Input: part model. Units: mm. Frame: model coordinates. A direction names the side the tool comes from. Give positions to 0.01 mm unless a question says otherwise; leave off trailing zeros. Loops run counter-clockwise (first coordinate to the right, second up) from the corner with the lowest first, then second, coordinate; pieces in that order, holes last. Notation, with made-up numbers: (52.25, 13.25) - (85.25, 13.25) arc R19 ccw to (85.25, 41.25) - close; hole circle Ø10 at (88, 59.5). An arc over 180 degrees is marked (long way). Answer as a JSON object with one key per item and string values.
from build123d import *

# Parameters (mm, degrees)
SKETCH1_W           = 25
SKETCH1_H           = 12
SKETCH1_R           = 1.5
BOSS_EXTRUDE1_DEPTH = 1
SKETCH2_R           = 1.5
SKETCH2_R_2         = 1
BOSS_EXTRUDE2_DEPTH = 6.25
BOSS_EXTRUDE3_START = 12.5
SKETCH3_R           = 1.5
SKETCH3_R_2         = 1
BOSS_EXTRUDE3_DEPTH = 6.25


with BuildPart() as part:
    # Sketch1 → Boss-Extrude1 (new body)
    with BuildSketch(Plane(origin=(0, 0, 0), x_dir=(1, 0, 0), z_dir=(0, 1, 0))):
        with Locations((12.5, 6)):
            Rectangle(SKETCH1_W, SKETCH1_H)
        with Locations((6, 6)):
            Circle(SKETCH1_R, mode=Mode.SUBTRACT)
        with Locations((19, 6)):
            Circle(SKETCH1_R, mode=Mode.SUBTRACT)
    extrude(amount=BOSS_EXTRUDE1_DEPTH)

    # Sketch2 → Boss-Extrude2 (add)
    with BuildSketch(Plane(origin=(0, 0, 0), x_dir=(0, 0, -1), z_dir=(1, 0, 0))):
        with Locations((-1, 1)):
            Circle(SKETCH2_R)
        with Locations((-1, 1)):
            Circle(SKETCH2_R_2, mode=Mode.SUBTRACT)
    extrude(amount=BOSS_EXTRUDE2_DEPTH)

    # Sketch3 → Boss-Extrude3 (add)
    with BuildSketch(Plane(origin=(0, 0, 0), x_dir=(0, 0, -1), z_dir=(1, 0, 0)).offset(BOSS_EXTRUDE3_START)):
        with Locations((-1, 1)):
            Circle(SKETCH3_R)
        with Locations((-1, 1)):
            Circle(SKETCH3_R_2, mode=Mode.SUBTRACT)
    extrude(amount=BOSS_EXTRUDE3_DEPTH)


solid = part.part
Item 1: Access query for faces 4 (the face through (21.8, 0.5, 0)), 5 (the face through (9.3, 0.5, 0)), 6 (the face through (12.3, 0.5, -12)). Directions: +Z, -Z, +X, -X, +Y, -Y. A direction counts if a zero-diameter tool reaches every point of the face in a straight line with its end or side. Return the directions, or none.
Geometry check:
{"face 4": "+Z, +X, +Y, -Y", "face 5": "+Z, +Y, -Y", "face 6": "-Z, +X, -X, +Y, -Y"}
Item 2: Contact query for flat-ended pins moving along their axis: P1, Ø6, axis at x = 11.5, z = -3.5, coming from the -Y side; P2, Ø1, axis at x = 21, y = 2, coming from the +Z side; P3, Ø1.5, axis at y = 0.5, z = 1, coming from the +X side; P4, Ø0.8, axis at x = 10.5, y = 0.5, coming from the +Z side. Output: stop coordinate, or through.
Geometry check:
{"P1": "stops at y = 0", "P2": "passes through", "P3": "stops at x = 18.75", "P4": "stops at z = 0"}
Item 3: Mould query, pull axis Y, two halves, no side actions, for faces 1 (the face through (3, 0, 1)), 2 (the face through (12, 1, -6)), 3 (the face through (17.5, 0.49, -6.07)). Classes: released by +Y, released by -Y, zero draft, split by the parting line, or undercut.
Geometry check:
{"face 1": "undercut", "face 2": "released by +Y", "face 3": "zero draft"}
Item 4: Cut plane C-C (z = -6). Return loops of the section in (x, y).
Geometry check:
{"outline": "(0, 0) - (4.5, 0) - (4.5, 1) - (0, 1) - close; (7.5, 0) - (17.5, 0) - (17.5, 1) - (7.5, 1) - close; (20.5, 0) - (25, 0) - (25, 1) - (20.5, 1) - close"}
Item 5: Cut plane B-B (x = 5.5). Return loops of the section in (y, z), then the cut area to 3 significant figures.
Geometry check:
{"outline": "(0, -12) - (1, -12) - (1, -7.41) - (0, -7.41) - close; (0, -4.59) - (1, -4.59) - (1, -0.5) arc R1.5 ccw (long way) to (0, -0.12) - close; hole circle Ø2 at (1, 1)", "area": "12.7 mm2"}
Item 6: Cut plane A-A (z = 1). Return loops of the section in (x, y), then the cut area to 3 significant figures.
Geometry check:
{"outline": "(0, -0.5) - (6.25, -0.5) - (6.25, 0) - (0, 0) - close; (0, 2) - (6.25, 2) - (6.25, 2.5) - (0, 2.5) - close; (12.5, -0.5) - (18.75, -0.5) - (18.75, 0) - (12.5, 0) - close; (12.5, 2) - (18.75, 2) - (18.75, 2.5) - (12.5, 2.5) - close", "area": "12.5 mm2"}
Item 7: Cut plane D-D (y = 1.7). Return loops of the section in (x, z), then the cut area to 3 significant figures.
Geometry check:
{"outline": "(0, -0.33) - (6.25, -0.33) - (6.25, 0.29) - (0, 0.29) - close; (0, 1.71) - (6.25, 1.71) - (6.25, 2.33) - (0, 2.33) - close; (12.5, -0.33) - (18.75, -0.33) - (18.75, 0.29) - (12.5, 0.29) - close; (12.5, 1.71) - (18.75, 1.71) - (18.75, 2.33) - (12.5, 2.33) - close", "area": "15.3 mm2"}
Item 8: Material intervals for line 1 (X direction, y = 0.4, z = -6); line 2 (Z direction, x = 6, y = 0.45); line 3 (Z direction, x = 19, y = 0.7), sorted ascending. Write a range as [from, to].
Geometry check:
{"line 1": "x = [0, 4.5], [7.5, 17.5], [20.5, 25]", "line 2": "z = [-12, -7.5], [-4.5, 0.16], [1.84, 2.4]", "line 3": "z = [-12, -7.5], [-4.5, 0]"}
